Source: CAD feature listing. Evaluate the final solid. Frame: model axes, mm. Face numbers are marked on the shaded views. A direction names the side the tool comes from. Coordinates: 2 decimals unless noted, no trailing zeros. Order: outer loops, then holes, each group sorted by start corner. A loop starts at its lowest first (then second) coordinate and runs counter-clockwise, first axis right, second up.
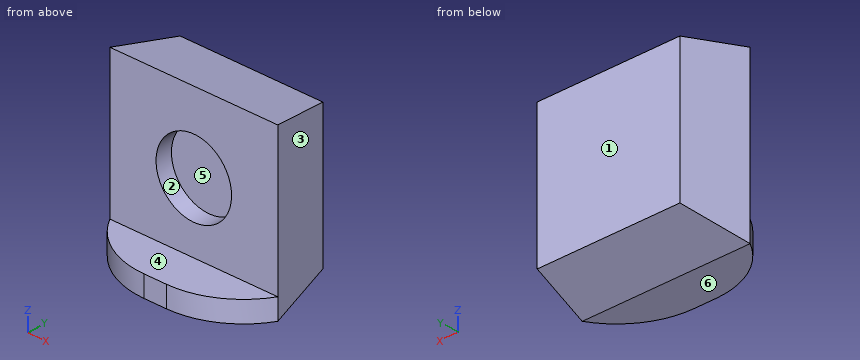
```python
from build123d import *

# Parameters (mm, degrees)
SKETCH1_W               = 8
SKETCH1_H               = 8
BOSS_EXTRUDE1_DEPTH     = 3
CUT_EXTRUDE1_DEPTH      = 12.704699911
CUT_EXTRUDE1_DEPTH_BACK = 12.704699911
CUT_EXTRUDE2_DEPTH      = 11
SKETCH4_R               = 1.8
CUT_EXTRUDE3_DEPTH      = 0.8
SKETCH5_W               = 8
SKETCH5_H               = 1
BOSS_EXTRUDE2_DEPTH     = 2
FILLET1_R               = 4


with BuildPart() as part:
    # Sketch1 → Boss-Extrude1 (new body)
    with BuildSketch(Plane(origin=(0, 0, 0), x_dir=(1, 0, 0), z_dir=(0, 1, 0))):
        with Locations((4, 4)):
            Rectangle(SKETCH1_W, SKETCH1_H)
    extrude(amount=BOSS_EXTRUDE1_DEPTH)

    # Sketch2 → Cut-Extrude1 (cut, two sides: drawn at the far end of the back side and taken through both)
    with BuildSketch(Plane.XY.offset(-CUT_EXTRUDE1_DEPTH_BACK)):
        Polygon((0, 0), (0.6, 3), (0, 3), align=None)
        Polygon((8, 0), (7.4, 3), (8, 3), align=None)
    extrude(amount=CUT_EXTRUDE1_DEPTH + CUT_EXTRUDE1_DEPTH_BACK, mode=Mode.SUBTRACT)

    # Sketch3 → Cut-Extrude2 (cut)
    with BuildSketch(Plane(origin=(0, 0, 0), x_dir=(0, 0, -1), z_dir=(1, 0, 0))):
        Polygon((0, 0), (0.6, 3), (0, 3), align=None)
        Polygon((8, 3), (7.4, 3), (8, 0), align=None)
    extrude(amount=CUT_EXTRUDE2_DEPTH, mode=Mode.SUBTRACT)

    # Sketch4 → Cut-Extrude3 (cut)
    with BuildSketch(Plane.XZ):
        with Locations(Location((4, -3.75, 0), (0, 0, 270))):
            Circle(SKETCH4_R)
    extrude(amount=-CUT_EXTRUDE3_DEPTH, mode=Mode.SUBTRACT)

    # Sketch5 → Boss-Extrude2 (add)
    with BuildSketch(Plane.XZ):
        with Locations((4, -7.5)):
            Rectangle(SKETCH5_W, SKETCH5_H)
    extrude(amount=BOSS_EXTRUDE2_DEPTH)

    # Fillet1
    # the kernel refuses this fillet: 4 mm, written as the material it takes off along each edge
    with BuildSketch(Plane(origin=(8, -2, -16.660254038), x_dir=(0, 1, 0), z_dir=(0, 0, 1)), Plane(origin=(0, -2, 1.660254038), x_dir=(0, 1, 0), z_dir=(0, 0, -1))) as fillet1_piece_1:
        with BuildLine():
            CenterArc((4, 3.464101615), FILLET1_R, 180, 60)
            Line((0, 3.464101615), (-0.08, 3.464101615))
            Line((-0.08, 3.464101615), (-0.08, 0))
            Line((-0.08, 0), (0, -0.08))
            ThreePointArc((0, -0.08), (1, -0.08), (1.96, -0.069282032))
            Line((1.96, -0.069282032), (2, 0))
        make_face()
    extrude(amount=18.320508076, mode=Mode.SUBTRACT)


solid = part.part
```
1. Draft query along X for the marked faces 1, 2 and 3. Return one class per face: released by +X, released by -X, zero draft, split by the parting line, or undercut.
Findings:
face 1: zero draft
face 2: undercut
face 3: released by +X
2. Access query for the marked faces 4, 5 and 6. Directions: +Z, -Z, +X, -X, +Y, -Y. A direction counts if a zero-diameter tool reaches every point of the face in a straight line with its end or side. Return the directions, or none.
Findings:
face 4: +Z, +X, -X, -Y
face 5: -Y
face 6: -Z, +X, -X, +Y, -Y
3. Ray query, line 1 (Y direction, x = 1, z = -6.25); line 2 (Z direction, x = 5.5, y = -1); line 3 (Y direction, x = 3, z = -2.75). Return the intervals inside material, ascending.
Findings:
line 1: y = 0 to 3
line 2: z = -8 to -7
line 3: y = 0.8 to 3
4. Section query C-C on y = 0.55. Return loops of the section in (x, z), plus the area to 3 significant figures.
Findings:
outline: (0.11, -7.89) - (7.89, -7.89) - (7.89, -0.11) - (0.11, -0.11) - close; hole circle Ø3.6 at (4, -3.75)
area: 50.3 mm2
5. Section query D-D on y = 1.85. Return loops of the section in (x, z), plus the area to 3 significant figures.
Findings:
outline: (0.37, -7.63) - (7.63, -7.63) - (7.63, -0.37) - (0.37, -0.37) - close
area: 52.7 mm2
6. Section query A-A on z = -3.75. Return loops of the section in (x, y).
Findings:
outline: (0, 0) - (2.2, 0) - (2.2, 0.8) - (5.8, 0.8) - (5.8, 0) - (8, 0) - (7.4, 3) - (0.6, 3) - close
7. Section query B-B on x = 4. Return loops of the section in (y, z), plus the area to 3 significant figures.
Findings:
outline: (-2, -8) - (0, -8) - (3, -7.4) - (3, -0.6) - (0, 0) - (0, -1.95) - (0.8, -1.95) - (0.8, -5.55) - (0, -5.55) - (0, -7) - (-2, -7) - close
area: 21.3 mm2
8. Pin query (flat end, axial travel): P1, Ø1, axis at x = 4.5, y = -1, coming from the +Z side; P2, Ø2, axis at x = 3, z = -4.5, coming from the -Y side; P3, Ø3, axis at x = 4, z = -3.75, coming from the -Y side. Return the tip coordinate at first contact, or that it passes through.
Findings:
P1: stops at z = -7
P2: stops at y = 0
P3: stops at y = 0.8
